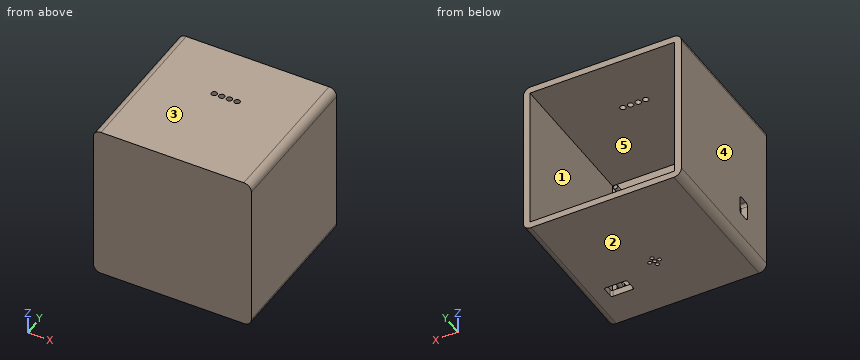
from build123d import *

# Parameters (mm, degrees)
SKETCH4_W                = 83
SKETCH4_H                = 83
BOSS_EXTRUDE2_DEPTH      = 40
BOSS_EXTRUDE2_DEPTH_BACK = 40
SKETCH5_W                = 76
SKETCH5_H                = 76
CUT_EXTRUDE1_DEPTH       = 50
CUT_EXTRUDE1_DEPTH_BACK  = 37.5
SKETCH6_R                = 1.5
CUT_EXTRUDE2_DEPTH       = 74.5
CUT_EXTRUDE2_DEPTH_BACK  = 5
SKETCH8_R                = 1
CUT_EXTRUDE3_DEPTH       = 70.5
SKETCH9_W                = 12
SKETCH9_H                = 7
CUT_EXTRUDE4_DEPTH       = 108.5
FILLET2_R                = 1
FILLET3_R                = 4
SKETCH10_W               = 10
SKETCH10_H               = 7
CUT_EXTRUDE5_DEPTH       = 83
FILLET4_R                = 1.5
SKETCH11_R               = 2
BOSS_EXTRUDE4_DEPTH      = 5
SKETCH12_R               = 1.2
BOSS_EXTRUDE5_DEPTH      = 10


with BuildPart() as part:
    # Sketch4 → Boss-Extrude2 (new body, two sides)
    with BuildSketch(Plane(origin=(0, 0, 0), x_dir=(1, 0, 0), z_dir=(0, 1, 0))) as boss_extrude2_sk:
        Rectangle(SKETCH4_W, SKETCH4_H)
    extrude(amount=BOSS_EXTRUDE2_DEPTH)
    extrude(boss_extrude2_sk.sketch, amount=-BOSS_EXTRUDE2_DEPTH_BACK)

    # Sketch5 → Cut-Extrude1 (cut, two sides)
    with BuildSketch(Plane(origin=(0, 0, 0), x_dir=(1, 0, 0), z_dir=(0, 1, 0))) as cut_extrude1_sk:
        Rectangle(SKETCH5_W, SKETCH5_H)
    extrude(amount=CUT_EXTRUDE1_DEPTH, mode=Mode.SUBTRACT)
    extrude(cut_extrude1_sk.sketch, amount=-CUT_EXTRUDE1_DEPTH_BACK, mode=Mode.SUBTRACT)

    # Sketch6 → Cut-Extrude2 (cut, two sides)
    with BuildSketch(Plane.XY) as cut_extrude2_sk:
        with Locations((2, 10)):
            Circle(SKETCH6_R)
        with Locations((6, 10)):
            Circle(SKETCH6_R)
        with Locations((-2, 10)):
            Circle(SKETCH6_R)
        with Locations((-6, 10)):
            Circle(SKETCH6_R)
    extrude(amount=CUT_EXTRUDE2_DEPTH, mode=Mode.SUBTRACT)
    extrude(cut_extrude2_sk.sketch, amount=-CUT_EXTRUDE2_DEPTH_BACK, mode=Mode.SUBTRACT)

    # Sketch8 → Cut-Extrude3 (cut)
    with BuildSketch(Plane.XY):
        with Locations((0, -9)):
            Circle(SKETCH8_R)
        with Locations((2.5, -9)):
            Circle(SKETCH8_R)
        with Locations((0, -6.5)):
            Circle(SKETCH8_R)
        with Locations((-2.5, -9)):
            Circle(SKETCH8_R)
        with Locations((0, -11.5)):
            Circle(SKETCH8_R)
    extrude(amount=-CUT_EXTRUDE3_DEPTH, mode=Mode.SUBTRACT)

    # Sketch9 → Cut-Extrude4 (cut)
    with BuildSketch(Plane.XY):
        with Locations((24, -18.5)):
            Rectangle(SKETCH9_W, SKETCH9_H)
    extrude(amount=-CUT_EXTRUDE4_DEPTH, mode=Mode.SUBTRACT)

    # Fillet2
    fillet2_edges = [part.edges().sort_by_distance(p)[0] for p in [
        (18, -22, -39.75),
        (18, -15, -39.75),
        (30, -15, -39.75),
        (30, -22, -39.75),
    ]]
    fillet(fillet2_edges, radius=FILLET2_R)

    # Fillet3
    fillet3_edges = [part.edges().sort_by_distance(p)[0] for p in [
        (-41.5, 0, -41.5),
        (41.5, 0, -41.5),
        (41.5, 0, 41.5),
        (-41.5, 0, 41.5),
    ]]
    fillet(fillet3_edges, radius=FILLET3_R)

    # Sketch10 → Cut-Extrude5 (cut)
    with BuildSketch(Plane(origin=(0, 0, 0), x_dir=(0, 0, -1), z_dir=(1, 0, 0))):
        with Locations((20, -18.5)):
            Rectangle(SKETCH10_W, SKETCH10_H)
    extrude(amount=-CUT_EXTRUDE5_DEPTH, mode=Mode.SUBTRACT)

    # Fillet4
    fillet4_edges = [part.edges().sort_by_distance(p)[0] for p in [
        (-39.75, -22, -15),
        (-39.75, -15, -15),
        (-39.75, -15, -25),
        (-39.75, -22, -25),
    ]]
    fillet(fillet4_edges, radius=FILLET4_R)

    # Sketch11 → Boss-Extrude4 (add)
    with BuildSketch(Plane(origin=(0, -37.5, 0), x_dir=(1, 0, 0), z_dir=(0, 1, 0))):
        with Locations((30.875, 27.5)):
            Circle(SKETCH11_R)
        with Locations((-30.875, 27.5)):
            Circle(SKETCH11_R)
        with Locations((-30.875, -27.5)):
            Circle(SKETCH11_R)
        with Locations((30.875, -27.5)):
            Circle(SKETCH11_R)
    extrude(amount=BOSS_EXTRUDE4_DEPTH)

    # Sketch12 → Boss-Extrude5 (add)
    with BuildSketch(Plane(origin=(0, -37.5, 0), x_dir=(1, 0, 0), z_dir=(0, 1, 0))):
        with Locations((-30.875, 27.5)):
            Circle(SKETCH12_R)
        with Locations((30.875, 27.5)):
            Circle(SKETCH12_R)
        with Locations((-30.875, -27.5)):
            Circle(SKETCH12_R)
        with Locations((30.875, -27.5)):
            Circle(SKETCH12_R)
    extrude(amount=BOSS_EXTRUDE5_DEPTH)


solid = part.part
CAD build for the part. Positions are in the model's coordinates, mm. Face numbers are marked on the shaded views. A direction names the side the tool comes from. Give positions to 0.01 mm unless a question says otherwise; leave off trailing zeros. Loops run counter-clockwise (first coordinate to the right, second up) from the corner with the lowest first, then second, coordinate; pieces in that order, holes last. Notation, with made-up numbers: M -35.75,31 L 4.25,31 A20 cw 4.25,58 Z; hole C -20.75,29 d1. An arc over 180 degrees is marked long. One line per question, with ' | ' between items. Start each with the question number.
1. Saw through at B-B on z = -18.5. Give the cut face in (x, y).
2. Saw through at C-C on y = 10. Give the cut face in (x, z).
3. Saw through at A-A on x = 6. Give the cut face in (y, z), plus the area to 4 significant figures.
4. Probe L1, parallel to Y at x = 0, z = -39.2; L2, parallel to Y at x = -6, z = 39; L3, parallel to Y at x = 2.5, z = -40. List the from-to ranges inside material, lowest first. Write a range as from..to.
5. 3-axis set-ups, long thin cutter, end or side, ignore diameter. For the marked faces 4 and 5: which of +Z, -Z, +X, -X, +Y, -Y reach the whole face in a straight line?
6. Flat gauge pins, fed straight in: pin 1 (10 mm diameter, centred on x = -1.5, z = 8, fed in from +Y); pin 2 (2 mm diameter, centred on x = -31, z = -27, fed in from +Y); pin 3 (1.2 mm diameter, centred on x = 0, y = -6.5, fed in from -Z). Where does each tip first touch, or does it go through?
7. Two-plate mould, pull along Z, no slides. Class the marked faces 1, 2 and 3: pulls with the +Z half, pulls with the -Z half, needs draft (parallel to the pull), parting line crosses it, or undercut.
8. Saw through at D-D on z = -27.5. Give the cut face in (x, y) (3 decimals).
Result sheet:
1) outline: M -41.5,-40 L 41.5,-40 L 41.5,40 L 38,40 L 38,-37.5 L -38,-37.5 L -38,-22 L -41.5,-22 Z; M -41.5,-15 L -38,-15 L -38,40 L -41.5,40 Z
2) outline: M -41.5,-37.5 A4 ccw -37.5,-41.5 L 37.5,-41.5 A4 ccw 41.5,-37.5 L 41.5,37.5 A4 ccw 37.5,41.5 L 7.5,41.5 L 7.5,38 L 38,38 L 38,-38 L -38,-38 L -38,38 L -7.5,38 L -7.5,41.5 L -37.5,41.5 A4 ccw -41.5,37.5 Z; M -4.5,38 L -3.5,38 L -3.5,41.5 L -4.5,41.5 Z; M -0.5,38 L 0.5,38 L 0.5,41.5 L -0.5,41.5 Z; M 3.5,38 L 4.5,38 L 4.5,41.5 L 3.5,41.5 Z
3) outline: M -40,-41.5 L 40,-41.5 L 40,-38 L -37.5,-38 L -37.5,38 L 8.5,38 L 8.5,41.5 L -40,41.5 Z; M 11.5,38 L 40,38 L 40,41.5 L 11.5,41.5 Z | area: 739.5 mm^2
4) L1: y = -40..-12.5, -10.5..-10, -8..-7.5, -5.5..40 | L2: y = -40..8.5, 11.5..40 | L3: y = -40..-10, -8..40
5) face 4: +Z, -Z, -X, +Y, -Y | face 5: +Y
6) pin 1: stops at y = -37.5 | pin 2: stops at y = -27.5 | pin 3: stops at z = 38
7) face 1: undercut | face 2: pulls with the -Z half | face 3: pulls with the +Z half
8) outline: M -41.5,-40 L 41.5,-40 L 41.5,40 L 38,40 L 38,-37.5 L 32.875,-37.5 L 32.875,-32.5 L 32.075,-32.5 L 32.075,-27.5 L 29.675,-27.5 L 29.675,-32.5 L 28.875,-32.5 L 28.875,-37.5 L -28.875,-37.5 L -28.875,-32.5 L -29.675,-32.5 L -29.675,-27.5 L -32.075,-27.5 L -32.075,-32.5 L -32.875,-32.5 L -32.875,-37.5 L -38,-37.5 L -38,40 L -41.5,40 Z
